The listing builds one solid part. Answer for the finished solid, in the listing's coordinates (mm). Round coordinates to 2 decimals unless told otherwise and drop trailing zeros. Order: outer loops, then holes, each group sorted by start corner. A loop starts at its lowest first (then second) coordinate and runs counter-clockwise, first axis right, second up. Notation, with made-up numbers: (-29, -6.5) - (20, -6.5) arc R18 ccw to (20, 22.5) - close; hole circle Ø7 at (82, 10.25). An arc over 180 degrees is marked (long way). Write item = value, one per line.
from build123d import *

# Parameters (mm, degrees)
SKETCH1_R           = 2.350480947
BOSS_EXTRUDE1_DEPTH = 1.5
CUT_EXTRUDE1_REACH  = 52.196
SKETCH2_R           = 2.5


with BuildPart() as part:
    # Sketch1 → Boss-Extrude1 (new body)
    with BuildSketch(Plane.XY):
        Polygon((-22.5, 29.75), (-22.5, -29.75), (22.5, -29.75), (22.5, 29.75), (22.5, 44.846109292), (-22.5, 44.846109292), align=None)
        with Locations((-17.503755709, 17.495628345)):
            Circle(SKETCH1_R, mode=Mode.SUBTRACT)
        with Locations((17.496244291, 17.495628345)):
            Circle(SKETCH1_R, mode=Mode.SUBTRACT)
        with Locations((17.496244291, -17.504371655)):
            Circle(SKETCH1_R, mode=Mode.SUBTRACT)
        with Locations((-17.5, -17.5)):
            Circle(SKETCH1_R, mode=Mode.SUBTRACT)
    extrude(amount=BOSS_EXTRUDE1_DEPTH)

    # Sketch2 → Cut-Extrude1 (cut, up to next)
    with BuildSketch(Plane.XY.offset(1.5), mode=Mode.PRIVATE) as cut_extrude1_sk1:
        with Locations((-15, 34.846109292)):
            Circle(SKETCH2_R)
    cut_extrude1_tool1 = extrude(cut_extrude1_sk1.sketch, amount=-CUT_EXTRUDE1_REACH, mode=Mode.PRIVATE) & part.part
    # Sketch2 → Cut-Extrude1 (cut, up to next)
    with BuildSketch(Plane.XY.offset(1.5), mode=Mode.PRIVATE) as cut_extrude1_sk2:
        with Locations((0, 34.846109292)):
            Circle(SKETCH2_R)
    cut_extrude1_tool2 = extrude(cut_extrude1_sk2.sketch, amount=-CUT_EXTRUDE1_REACH, mode=Mode.PRIVATE) & part.part
    # Sketch2 → Cut-Extrude1 (cut, up to next)
    with BuildSketch(Plane.XY.offset(1.5), mode=Mode.PRIVATE) as cut_extrude1_sk3:
        with Locations((15, 34.846109292)):
            Circle(SKETCH2_R)
    cut_extrude1_tool3 = extrude(cut_extrude1_sk3.sketch, amount=-CUT_EXTRUDE1_REACH, mode=Mode.PRIVATE) & part.part
    add(cut_extrude1_tool1.solids().sort_by_distance((-15, 34.846109, 1.5))[0], mode=Mode.SUBTRACT)
    add(cut_extrude1_tool2.solids().sort_by_distance((0, 34.846109, 1.5))[0], mode=Mode.SUBTRACT)
    add(cut_extrude1_tool3.solids().sort_by_distance((15, 34.846109, 1.5))[0], mode=Mode.SUBTRACT)


solid = part.part
Q1. Section A-A on x = 0 is taken. Determine the outline of the cut face in (y, z), then the cut area to 3 significant figures.
Model answer:
outline = (-29.75, 0) - (32.35, 0) - (32.35, 1.5) - (-29.75, 1.5) - close; (37.35, 0) - (44.85, 0) - (44.85, 1.5) - (37.35, 1.5) - close
area = 104 mm^2
Q2. Determine the mould class of faces 1 (the face through (-22.5, 8, 1)), 2 (the face through (0, 44.846, 1)), 3 (the face through (-15.26, 18.2, 0.74)) for opening direction Y: released by +Y, released by -Y, zero draft, split by the parting line, or undercut.
Model answer:
face_1 = zero draft
face_2 = released by +Y
face_3 = undercut
Q3. Section B-B on z = 0.4 is taken. Determine the outline of the cut face in (x, y).
Model answer:
outline = (-22.5, -29.75) - (22.5, -29.75) - (22.5, 44.85) - (-22.5, 44.85) - close; hole circle Ø4.7 at (-17.5, -17.5); hole circle Ø4.7 at (-17.5, 17.5); hole circle Ø5 at (-15, 34.85); hole circle Ø5 at (0, 34.85); hole circle Ø5 at (15, 34.85); hole circle Ø4.7 at (17.5, -17.5); hole circle Ø4.7 at (17.5, 17.5)
Q4. Find the intervals of material crossed by line 1 (Y direction, x = -16, z = 1.15); line 2 (X direction, y = 17, z = 0.3); line 3 (Y direction, x = 15, z = 0.65), in increasing order. Write a range as from..to.
Model answer:
line_1 = -29.75..-19.31, -15.69..15.69, 19.3..32.55, 37.14..44.85
line_2 = -22.5..-19.8, -15.21..15.2, 19.79..22.5
line_3 = -29.75..32.35, 37.35..44.85
Q5. Flat-ended cylindrical pins translate along their axes: P1, Ø6, axis at x = 17.5, y = -17.5, coming from the -Z side; P2, Ø3, axis at x = 0, y = 34.85, coming from the -Z side. Find the tip coordinate at first contact, or state that the pin passes through.
Model answer:
P1 = 0
P2 = through
Q6. Section C-C on y = 19 is taken. Determine the outline of the cut face in (x, z).
Model answer:
outline = (-22.5, 0) - (-19.31, 0) - (-19.31, 1.5) - (-22.5, 1.5) - close; (-15.7, 0) - (15.69, 0) - (15.69, 1.5) - (-15.7, 1.5) - close; (19.3, 0) - (22.5, 0) - (22.5, 1.5) - (19.3, 1.5) - close
